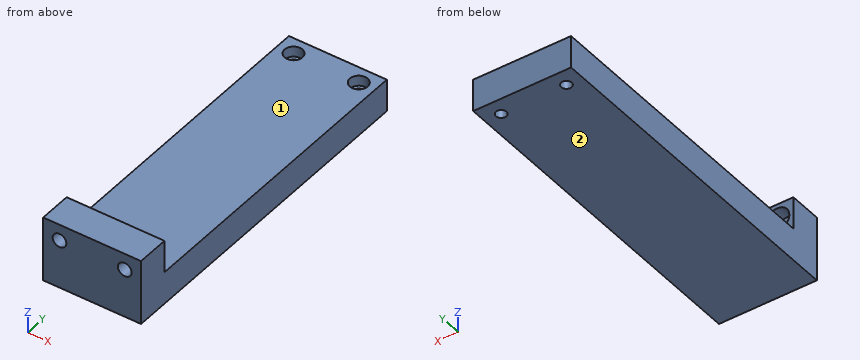
from build123d import *

# Parameters (mm, degrees)
SKETCH_2_W                   = 60
SKETCH_2_H                   = 210
EXTRUDE_1_DEPTH              = 40
SKETCH_3_W                   = 60
SKETCH_3_H                   = 190
CUT_EXTRUDE_1_DEPTH          = 20
HOLE_WIZARD_M6_2_D           = 6.4
HOLE_WIZARD_M6_2_CBORE_D     = 11
HOLE_WIZARD_M6_2_CBORE_DEPTH = 6.4
HOLE_WIZARD_M8_2_D           = 8.4
HOLE_WIZARD_M8_2_CBORE_D     = 15
HOLE_WIZARD_M8_2_CBORE_DEPTH = 8.6


with BuildPart() as part:
    # 草图2 → 凸台-拉伸1 (new body)
    with BuildSketch(Plane.XY):
        Rectangle(SKETCH_2_W, SKETCH_2_H)
    extrude(amount=EXTRUDE_1_DEPTH)

    # 草图3 → 切除-拉伸1 (cut)
    with BuildSketch(Plane.XY.offset(40)):
        with Locations((0, 10)):
            Rectangle(SKETCH_3_W, SKETCH_3_H)
    extrude(amount=-CUT_EXTRUDE_1_DEPTH, mode=Mode.SUBTRACT)

    # M6 六角凹头螺钉的柱形沉头孔2 (through all)
    with Locations(Plane(origin=(-20, 95, 20), x_dir=(1, 0, 0), z_dir=(0, 0, 1))):
        with Locations((0, 0), (40, 0)):
            CounterBoreHole(HOLE_WIZARD_M6_2_D / 2, HOLE_WIZARD_M6_2_CBORE_D / 2, HOLE_WIZARD_M6_2_CBORE_DEPTH)

    # M8 六角凹头螺钉的柱形沉头孔2 (through all)
    with Locations(Plane(origin=(-20, -85, 30), x_dir=(0, 0, 1), z_dir=(0, 1, 0))):
        with Locations((0, 0), (0, 40)):
            CounterBoreHole(HOLE_WIZARD_M8_2_D / 2, HOLE_WIZARD_M8_2_CBORE_D / 2, HOLE_WIZARD_M8_2_CBORE_DEPTH)


solid = part.part
Verification items for the finished model (mm, model axes). Face numbers are marked on the shaded views. A direction names the side the tool comes from. Give positions to 0.01 mm unless a question says otherwise; leave off trailing zeros. Loops run counter-clockwise (first coordinate to the right, second up) from the corner with the lowest first, then second, coordinate; pieces in that order, holes last.
1. Cross-section at B-B on y = 95. Record the cut outline in (x, z), and give its area (3 significant figures).
Derived:
outline: (-30, 0) - (-23.2, 0) - (-23.2, 13.6) - (-25.5, 13.6) - (-25.5, 20) - (-30, 20) - close; (-16.8, 0) - (16.8, 0) - (16.8, 13.6) - (14.5, 13.6) - (14.5, 20) - (-14.5, 20) - (-14.5, 13.6) - (-16.8, 13.6) - close; (23.2, 0) - (30, 0) - (30, 20) - (25.5, 20) - (25.5, 13.6) - (23.2, 13.6) - close
area: 885 mm2
2. Cross-section at A-A on z = 30. Record the cut outline in (x, y), and give its area (3 significant figures).
Derived:
outline: (-30, -105) - (-24.2, -105) - (-24.2, -93.6) - (-27.5, -93.6) - (-27.5, -85) - (-30, -85) - close; (-15.8, -105) - (15.8, -105) - (15.8, -93.6) - (12.5, -93.6) - (12.5, -85) - (-12.5, -85) - (-12.5, -93.6) - (-15.8, -93.6) - close; (24.2, -105) - (30, -105) - (30, -85) - (27.5, -85) - (27.5, -93.6) - (24.2, -93.6) - close
area: 750 mm2
3. Cross-section at D-D on x = 10. Record the cut outline in (y, z).
Derived:
outline: (-105, 0) - (105, 0) - (105, 20) - (-85, 20) - (-85, 40) - (-105, 40) - close
4. Tool access check on the marked faces 1 and 2. Record the directions out of +Z, -Z, +X, -X, +Y, -Y that give a thin tool (end or side, any length) a straight path to the whole face; none if there is none.
Derived:
face 1: +Z, +X, -X, +Y
face 2: -Z, +X, -X, +Y, -Y
5. Cross-section at C-C on x = 20. Record the cut outline in (y, z), and give its area (3 significant figures).
Derived:
outline: (-105, 0) - (91.8, 0) - (91.8, 13.6) - (89.5, 13.6) - (89.5, 20) - (-85, 20) - (-85, 22.5) - (-93.6, 22.5) - (-93.6, 25.8) - (-105, 25.8) - close; (-105, 34.2) - (-93.6, 34.2) - (-93.6, 37.5) - (-85, 37.5) - (-85, 40) - (-105, 40) - close; (98.2, 0) - (105, 0) - (105, 20) - (100.5, 20) - (100.5, 13.6) - (98.2, 13.6) - close
area: 4,220 mm2
6. Material ranges on probe 1 along X at (y, z) = (-88.5, 30); probe 2 along X at (y, z) = (-100, 30); probe 3 along Y at (x, z) = (-20, 11.25), recorded low to high.
Derived:
probe 1: x = -30 to -27.5, -12.5 to 12.5, 27.5 to 30
probe 2: x = -30 to -24.2, -15.8 to 15.8, 24.2 to 30
probe 3: y = -105 to 91.8, 98.2 to 105
7. Go/stop test with flat-tipped pins: P1, Ø8.5, axis at x = 20, y = 95, coming from the +Z side; P2, Ø7.5, axis at x = -18.5, z = 31, coming from the +Y side; P3, Ø12, axis at x = -18.5, y = 93, coming from the +Z side. Record where each tip stops, or that it passes through.
Derived:
P1: stops at z = 13.6
P2: stops at y = -93.6
P3: stops at z = 20
